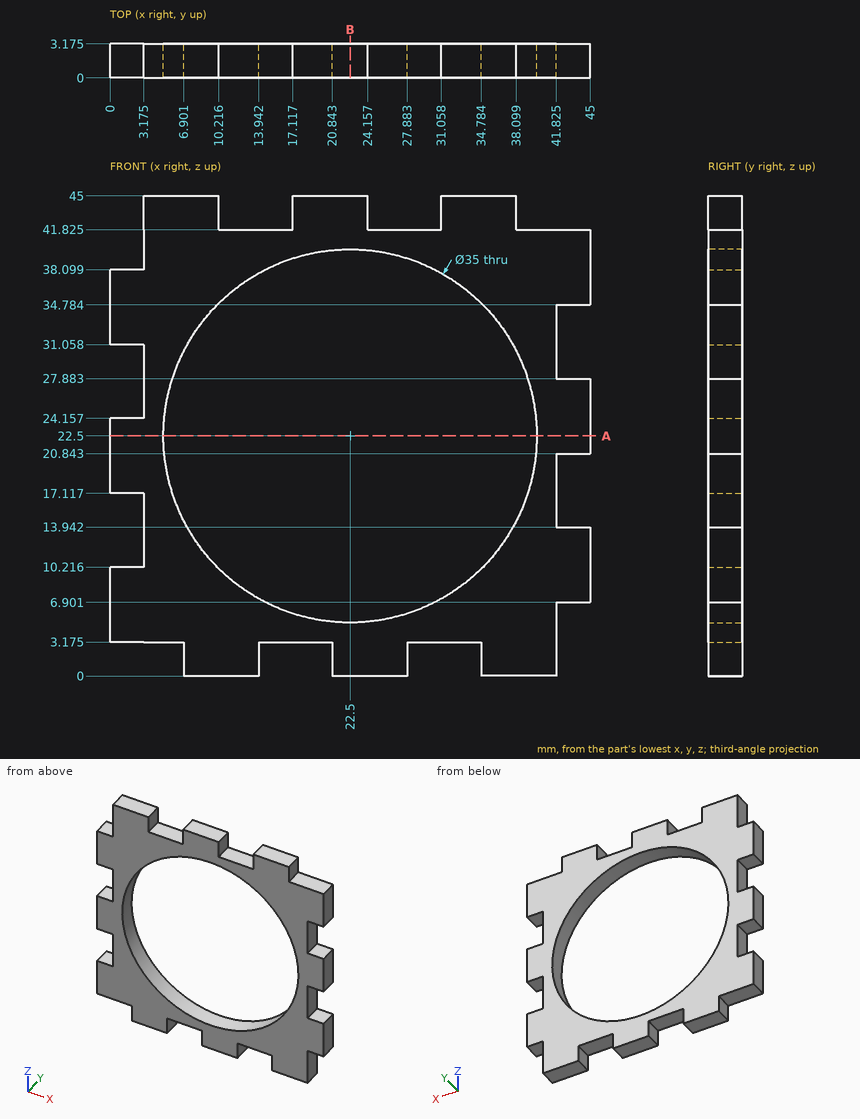
Verification items for this drawing (mm, ordinates from the low corner). Give positions to 0.01 mm unless a question says otherwise; leave off trailing zeros. Loops run counter-clockwise (first coordinate to the right, second up) from the corner with the lowest first, then second, coordinate; pieces in that order, holes last. Notation, with made-up numbers: M -19.5,55 L 9.5,55 A24 cw 9.5,81 Z; hole C -40,47 d2. An arc over 180 degrees is marked long. Answer as a JSON object with one key per item and string values. Group by question number.
Item 1: Gauge pin test, flat ends, axial feed: pin 1 (1 mm diameter, centred on y = 2, z = 43.5, fed in from -X) (1 decimal); pin 2 (1.6 mm diameter, centred on x = 2, y = 1.5, fed in from +Z); pin 3 (1.6 mm diameter, centred on x = 43, y = 1.5, fed in from +Z) (1 decimal). Record the tip position at first contact, or that the pin passes through.
Item 2: Sectioned sample at B-B on x = 22.5. Record the boundary of the cut face in (y, z) (1 decimal).
Item 3: Sectioned sample at A-A on z = 22.5. Record the boundary of the cut face in (x, y) (1 decimal).
Item 4: Material ranges on L1, parallel to X at y = 1.5, z = 22.5; L2, parallel to Z at x = 2, y = 2.55 (1 decimal), recorded low to high.
Findings below:
{
 "1": {"pin 1": "x = 3.2", "pin 2": "z = 38.1", "pin 3": "z = 41.8"},
 "2": {"outline": "M 0,0 L 3.2,0 L 3.2,5 L 0,5 Z; M 0,40 L 3.2,40 L 3.2,45 L 0,45 Z"},
 "3": {"outline": "M 0,0 L 5,0 L 5,3.2 L 0,3.2 Z; M 40,0 L 45,0 L 45,3.2 L 40,3.2 Z"},
 "4": {"L1": "0 to 5, 40 to 45", "L2": "3.2 to 10.2, 17.1 to 24.2, 31.1 to 38.1"}
}
